from build123d import *

# Parameters (mm, degrees)
F1_DEPTH = 203.2
F2_DEPTH = 25.4


with BuildPart() as f1:
    # F0 (on Front) → F1 (new body)
    with BuildSketch(Plane.XZ):
        with BuildLine():
            ThreePointArc((0, -44.45), (-44.45, 0), (0, 44.45))
            Line((0, 44.45), (25.92662, 44.45))
            Line((25.92662, 44.45), (25.92662, 47.625))
            Line((25.92662, 47.625), (0, 47.625))
            ThreePointArc((0, 47.625), (-47.625, 0), (0, -47.625))
            Line((0, -47.625), (0, -44.45))
        make_face()
    extrude(amount=F1_DEPTH)

    # F0 (on Front) → F2 (join)
    with BuildSketch(Plane.XZ):
        with BuildLine():
            ThreePointArc((0, -44.45), (-44.45, 0), (0, 44.45))
            Line((0, 44.45), (25.92662, 44.45))
            Line((25.92662, 44.45), (25.92662, 47.625))
            Line((25.92662, 47.625), (0, 47.625))
            ThreePointArc((0, 47.625), (-47.625, 0), (0, -47.625))
            Line((0, -47.625), (0, -44.45))
        make_face()
    extrude(amount=F2_DEPTH)


solid = f1.part
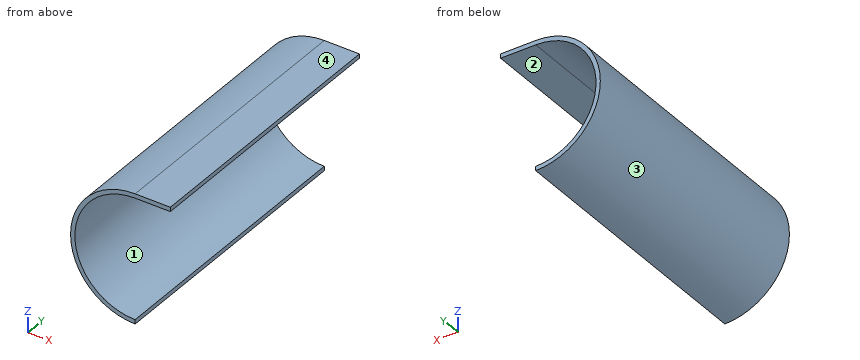
Check sheet for the modelled part. Datum: model origin and axes. Units: mm. Face numbers are marked on the shaded views. Round coordinates to 2 decimals unless told otherwise and drop trailing zeros. Write each loop counter-clockwise with the first axis right and the second up, starting at its lowest first coordinate (ties: lowest second). Pieces come first, ordered by that corner, then holes. Notation, with made-up numbers: (71, 27.25) - (81, 27.25) arc R16 cw to (81, 52.25) - close; hole circle Ø11 at (-38.5, 77). An arc over 180 degrees is marked (long way). Return JSON: item names as keys, results as strings.
Q1. Scan lines: L1, parallel to Z at x = -1, y = -130; L2, parallel to X at y = -144, z = 0.5; L3, parallel to Z at x = 11, y = -89 (3 decimals). Record each from-to range of solid material in increasing order. Write a range as from..to.
Returned:
{"L1": "z = -47.61..-44.44, 44.44..47.61", "L2": "x = -47.62..-44.45", "L3": "z = 44.45..47.625"}
Q2. Cross-section at A-A (x = -29). Record the boundary of the cut face in (y, z), then the cut area to 3 significant figures.
Returned:
{"outline": "(-203.2, -37.78) - (0, -37.78) - (0, -33.69) - (-203.2, -33.69) - close; (-203.2, 33.69) - (0, 33.69) - (0, 37.78) - (-203.2, 37.78) - close", "area": "1,660 mm²"}
Q3. Draft check along Z on the marked faces 1, 2, 3 and 4. Enter one of: released by +Z, released by -Z, zero draft, split by the parting line, or undercut.
Returned:
{"face 1": "undercut", "face 2": "released by -Z", "face 3": "split by the parting line", "face 4": "released by +Z"}
Q4. Cross-section at C-C (x = 16). Record the boundary of the cut face in (y, z) (3 decimals), then the cut area to 3 significant figures.
Returned:
{"outline": "(-203.2, 44.45) - (0, 44.45) - (0, 47.625) - (-203.2, 47.625) - close", "area": "645 mm²"}
Q5. Depth check by flat-ended pin: P1, Ø4, axis at y = -146, z = -12, coming from the -X side; P2, Ø3.5, axis at y = -114.5, z = -46.5, coming from the +X side; P3, Ø10, axis at y = -35, z = -31.5, coming from the -X side. Enter the tip coordinate at first touch or a pass-through.
Returned:
{"P1": "stops at x = -46.56", "P2": "stops at x = 0", "P3": "stops at x = -39.57"}
Q6. Cross-section at B-B (y = -28.5). Record the boundary of the cut face in (x, z) (3 decimals).
Returned:
{"outline": "(0, -47.625) - (0, -44.45) arc R44.45 cw to (0, 44.45) - (25.927, 44.45) - (25.927, 47.625) - (0, 47.625) arc R47.625 ccw to start"}
Q7. Cross-section at D-D (z = 0). Record the boundary of the cut face in (x, y) (3 decimals), then the cut area to 3 significant figures.
Returned:
{"outline": "(-47.625, -203.2) - (-44.45, -203.2) - (-44.45, 0) - (-47.625, 0) - close", "area": "645 mm²"}
